Source: CAD feature listing. Evaluate the final solid. Frame: model axes, mm. A direction names the side the tool comes from. Coordinates: 2 decimals unless noted, no trailing zeros. Write each loop counter-clockwise with the first axis right and the second up, starting at its lowest first coordinate (ties: lowest second). Pieces come first, ordered by that corner, then holes. Notation, with made-up numbers: M 26,-31.5 L 73,-31.5 A18 ccw 73,-26.5 Z; hole C 34.25,17 d6. An arc over 180 degrees is marked long. Write item = value, one per line. Start each with the question number.
1. Access query for faces 5 (the face through (-40.52, 24.54, 33.99)), 6 (the face through (-40.52, 66.04, 33.99)), 7 (the face through (-36.61, 44.94, 34.79)), 8 (the face through (-91, 89, 30)), 9 (the face through (-100, 67, 30)). Directions: +Z, -Z, +X, -X, +Y, -Y. A direction counts if a zero-diameter tool reaches every point of the face in a straight line with its end or side. Return the directions, or none.
2. Pin query (flat end, axial travel): pin 1 Ø4 at (y, z) = (65, 25.5) entering from -X; pin 2 Ø10 at (x, y) = (-74, 22) entering from +Z; pin 3 Ø5 at (x, z) = (-90, 25.5) entering from +Y. Return the tip coordinate at first contact, or that it passes through.
3. Section query A-A (y = 10). Output: boundary loops of the cut face in (x, z).
4. Pull-direction query (Z, two-part tool) for faces 1 (the face through (-100.465, 30.344, 34.553)), 2 (the face through (-100, 28, 44.45)), 3 (the face through (-40, 68.5, 28)), 4 (the face through (-100.465, 25.776, 25.153)); classes: pulls with the +Z half, pulls with the -Z half, needs draft (parallel to the pull), parting line crosses it, or undercut.
5. Section query C-C (x = -100.5). Output: boundary loops of the cut face in (y, z).
6. Section query B-B (x = 10). Output: boundary loops of the cut face in (y, z).
7. Section query D-D (z = 24.45). Give the number of separate pieces and of enclosed holes in the cut face, then the cut area to 3 significant figures.
8. Line query: line 1 along Y through (x, z) = (10, 14.2); line 2 along Y through (x, z) = (-34, 31.5); line 3 along X through (y, z) = (87.75, 24.45). Output: solid intervals per line, ascending.
```python
from build123d import *

# Parameters (mm, degrees)
SKETCH169_R                = 2.34
EXTRUDE089_DEPTH           = 20
SKETCH168_W                = 10
SKETCH168_H                = 30
EXTRUDE088_DEPTH           = 5
EXTRUDE088_PLACEMENT_ANGLE = 90
CUT055_PLACEMENT_ANGLE     = 90
SKETCH165_R                = 2.34
EXTRUDE085_DEPTH           = 20
SKETCH164_W                = 10
SKETCH164_H                = 30
EXTRUDE084_DEPTH           = 5
EXTRUDE084_PLACEMENT_ANGLE = 90
SKETCH082_R                = 2.21
EXTRUDE103_DEPTH           = 10
SKETCH081_R                = 2.21
EXTRUDE102_DEPTH           = 10
SKETCH080_W                = 12
SKETCH080_H                = 26.01178
EXTRUDE101_DEPTH           = 5
SKETCH079_R                = 2.21
EXTRUDE100_DEPTH           = 10
SKETCH078_R                = 2.21
EXTRUDE099_DEPTH           = 10
SKETCH077_W                = 12
SKETCH077_H                = 26.01178
EXTRUDE098_DEPTH           = 5
SKETCH167_R                = 2.34
EXTRUDE087_DEPTH           = 20
SKETCH166_W                = 10
SKETCH166_H                = 30
EXTRUDE086_DEPTH           = 5
EXTRUDE086_PLACEMENT_ANGLE = 90
CUT052_PLACEMENT_ANGLE     = 90
SKETCH163_R                = 2.34
EXTRUDE083_DEPTH           = 20
SKETCH162_W                = 10
SKETCH162_H                = 30
EXTRUDE082_DEPTH           = 5
EXTRUDE082_PLACEMENT_ANGLE = 90
SKETCH016_R                = 2.005
EXTRUDE077_DEPTH           = 20
EXTRUDE076_DEPTH           = 20
EXTRUDE075_DEPTH           = 20
SKETCH161_W                = 10
SKETCH161_H                = 27.36
EXTRUDE182_DEPTH           = 70
SKETCH075_R                = 2.9
EXTRUDE091_DEPTH           = 50
SKETCH074_W                = 130
SKETCH074_H                = 90
EXTRUDE090_DEPTH           = 2


with BuildPart() as tornillos050:
    # Sketch169 (on Face6 of Extrude088) → Extrude089 (new body)
    with BuildSketch(Plane(origin=(-101, -107, 0), x_dir=(0, -1, 0), z_dir=(-1, 0, 0))):
        with Locations((-135.006037, 30)):
            Circle(SKETCH169_R)
        with Locations((-135.008375, 20)):
            Circle(SKETCH169_R)
    extrude(amount=EXTRUDE089_DEPTH)


with BuildPart() as tornillos050_1:
    # Extrude089 placement: moved
    add(tornillos050.part.moved(Location((17, 0, 0))))


with BuildPart() as soporte016:
    # Sketch168 → Extrude088 (new body)
    with BuildSketch(Plane.XZ):
        with Locations((-135, 25)):
            Rectangle(SKETCH168_W, SKETCH168_H)
    extrude(amount=EXTRUDE088_DEPTH)


with BuildPart() as soporte016_1:
    # Extrude088 placement: moved
    add(soporte016.part.moved(Location((-96, -107, 0))).rotate(Axis((-96, -107, 0), (0, 0, -1)), EXTRUDE088_PLACEMENT_ANGLE))

    # Cut055: cut Tornillos050
    add(tornillos050_1.part, mode=Mode.SUBTRACT)


with BuildPart() as soporte016_2:
    # Cut055 placement: moved
    add(soporte016_1.part.moved(Location((-119, -12, -3))).rotate(Axis((-119, -12, -3), (0, 0, -1)), CUT055_PLACEMENT_ANGLE))


with BuildPart() as tornillos048:
    # Sketch165 (on Face6 of Extrude084) → Extrude085 (new body)
    with BuildSketch(Plane(origin=(-101, -107, 0), x_dir=(0, -1, 0), z_dir=(-1, 0, 0))):
        with Locations((-135.006037, 30)):
            Circle(SKETCH165_R)
        with Locations((-135.008375, 20)):
            Circle(SKETCH165_R)
    extrude(amount=EXTRUDE085_DEPTH)


with BuildPart() as tornillos048_1:
    # Extrude085 placement: moved
    add(tornillos048.part.moved(Location((17, 0, 0))))


with BuildPart() as soporte015:
    # Sketch164 → Extrude084 (new body)
    with BuildSketch(Plane.XZ):
        with Locations((-135, 25)):
            Rectangle(SKETCH164_W, SKETCH164_H)
    extrude(amount=EXTRUDE084_DEPTH)


with BuildPart() as soporte015_1:
    # Extrude084 placement: moved
    add(soporte015.part.moved(Location((-96, -107, 0))).rotate(Axis((-96, -107, 0), (0, 0, -1)), EXTRUDE084_PLACEMENT_ANGLE))

    # Cut054: cut Tornillos048
    add(tornillos048_1.part, mode=Mode.SUBTRACT)


with BuildPart() as soporte015_2:
    # Cut054 placement: moved
    add(soporte015_1.part.moved(Location((-2, 34, -3))))


with BuildPart() as extrude103:
    # Sketch082 → Extrude103 (new body)
    with BuildSketch(Plane.XZ):
        with Locations((-30.242167, 20.01615)):
            Circle(SKETCH082_R)
    extrude(amount=EXTRUDE103_DEPTH)


with BuildPart() as extrude103_1:
    # Extrude103 placement: moved
    add(extrude103.part.moved(Location((-9.8, 5, -14.82))))


with BuildPart() as extrude102:
    # Sketch081 → Extrude102 (new body)
    with BuildSketch(Plane.XZ):
        with Locations((-30.242167, 20.01615)):
            Circle(SKETCH081_R)
    extrude(amount=EXTRUDE102_DEPTH)


with BuildPart() as extrude102_1:
    # Extrude102 placement: moved
    add(extrude102.part.moved(Location((-9.8, 3, 2.68))))


with BuildPart() as cut059:
    # Sketch080 → Extrude101 (new body)
    with BuildSketch(Plane.XZ):
        with Locations((-39.733391, 13.00589)):
            Rectangle(SKETCH080_W, SKETCH080_H)
    extrude(amount=EXTRUDE101_DEPTH)

    # Cut058: cut Extrude102
    add(extrude102_1.part, mode=Mode.SUBTRACT)

    # Cut059: cut Extrude103
    add(extrude103_1.part, mode=Mode.SUBTRACT)


with BuildPart() as cut059_1:
    # Cut059 placement: moved
    add(cut059.part.moved(Location((0, 68.5, 6))))


with BuildPart() as extrude100:
    # Sketch079 → Extrude100 (new body)
    with BuildSketch(Plane.XZ):
        with Locations((-30.242167, 20.01615)):
            Circle(SKETCH079_R)
    extrude(amount=EXTRUDE100_DEPTH)


with BuildPart() as extrude100_1:
    # Extrude100 placement: moved
    add(extrude100.part.moved(Location((-9.8, 5, -14.82))))


with BuildPart() as extrude099:
    # Sketch078 → Extrude099 (new body)
    with BuildSketch(Plane.XZ):
        with Locations((-30.242167, 20.01615)):
            Circle(SKETCH078_R)
    extrude(amount=EXTRUDE099_DEPTH)


with BuildPart() as extrude099_1:
    # Extrude099 placement: moved
    add(extrude099.part.moved(Location((-9.8, 3, 2.68))))


with BuildPart() as cut057:
    # Sketch077 → Extrude098 (new body)
    with BuildSketch(Plane.XZ):
        with Locations((-39.733391, 13.00589)):
            Rectangle(SKETCH077_W, SKETCH077_H)
    extrude(amount=EXTRUDE098_DEPTH)

    # Cut056: cut Extrude099
    add(extrude099_1.part, mode=Mode.SUBTRACT)

    # Cut057: cut Extrude100
    add(extrude100_1.part, mode=Mode.SUBTRACT)


with BuildPart() as cut057_1:
    # Cut057 placement: moved
    add(cut057.part.moved(Location((0, 27, 6))))


with BuildPart() as tornillos049:
    # Sketch167 (on Face6 of Extrude086) → Extrude087 (new body)
    with BuildSketch(Plane(origin=(-101, -107, 0), x_dir=(0, -1, 0), z_dir=(-1, 0, 0))):
        with Locations((-135.006037, 30)):
            Circle(SKETCH167_R)
        with Locations((-135.008375, 20)):
            Circle(SKETCH167_R)
    extrude(amount=EXTRUDE087_DEPTH)


with BuildPart() as tornillos049_1:
    # Extrude087 placement: moved
    add(tornillos049.part.moved(Location((17, 0, 0))))


with BuildPart() as soporte013:
    # Sketch166 → Extrude086 (new body)
    with BuildSketch(Plane.XZ):
        with Locations((-135, 25)):
            Rectangle(SKETCH166_W, SKETCH166_H)
    extrude(amount=EXTRUDE086_DEPTH)


with BuildPart() as soporte013_1:
    # Extrude086 placement: moved
    add(soporte013.part.moved(Location((-96, -107, 0))).rotate(Axis((-96, -107, 0), (0, 0, -1)), EXTRUDE086_PLACEMENT_ANGLE))

    # Cut052: cut Tornillos049
    add(tornillos049_1.part, mode=Mode.SUBTRACT)


with BuildPart() as soporte013_2:
    # Cut052 placement: moved
    add(soporte013_1.part.moved(Location((-119, -95, -3))).rotate(Axis((-119, -95, -3), (0, 0, -1)), CUT052_PLACEMENT_ANGLE))


with BuildPart() as tornillos047:
    # Sketch163 (on Face6 of Extrude082) → Extrude083 (new body)
    with BuildSketch(Plane(origin=(-101, -107, 0), x_dir=(0, -1, 0), z_dir=(-1, 0, 0))):
        with Locations((-135.006037, 30)):
            Circle(SKETCH163_R)
        with Locations((-135.008375, 20)):
            Circle(SKETCH163_R)
    extrude(amount=EXTRUDE083_DEPTH)


with BuildPart() as tornillos047_1:
    # Extrude083 placement: moved
    add(tornillos047.part.moved(Location((17, 0, 0))))


with BuildPart() as soporte014:
    # Sketch162 → Extrude082 (new body)
    with BuildSketch(Plane.XZ):
        with Locations((-135, 25)):
            Rectangle(SKETCH162_W, SKETCH162_H)
    extrude(amount=EXTRUDE082_DEPTH)


with BuildPart() as soporte014_1:
    # Extrude082 placement: moved
    add(soporte014.part.moved(Location((-96, -107, 0))).rotate(Axis((-96, -107, 0), (0, 0, -1)), EXTRUDE082_PLACEMENT_ANGLE))

    # Cut053: cut Tornillos047
    add(tornillos047_1.part, mode=Mode.SUBTRACT)


with BuildPart() as soporte014_2:
    # Cut053 placement: moved
    add(soporte014_1.part.moved(Location((-2, 0, -3))))


with BuildPart() as tornillo018:
    # Sketch016 → Extrude077 (new body)
    with BuildSketch(Plane.XY.offset(45.913223)):
        with Locations((-84.962639, 67.504814)):
            Circle(SKETCH016_R)
    extrude(amount=EXTRUDE077_DEPTH)


with BuildPart() as tornillo018_1:
    # Extrude077 placement: moved
    add(tornillo018.part.moved(Location((46.5, -21.8, -26))))


with BuildPart() as tornillo017:
    # Sketch016 → Extrude076 (new body)
    with BuildSketch(Plane.XY.offset(45.913223)):
        with Locations((-84.962639, 67.504814)):
            Circle(SKETCH016_R)
    extrude(amount=EXTRUDE076_DEPTH)


with BuildPart() as tornillo017_1:
    # Extrude076 placement: moved
    add(tornillo017.part.moved(Location((23.6, -21.8, -25.9))))


with BuildPart() as tornillo016:
    # Sketch016 → Extrude075 (new body)
    with BuildSketch(Plane.XY.offset(45.913223)):
        with Locations((-84.962639, 67.504814)):
            Circle(SKETCH016_R)
    extrude(amount=EXTRUDE075_DEPTH)


with BuildPart() as tornillo016_1:
    # Extrude075 placement: moved
    add(tornillo016.part.moved(Location((0, -21.8, -26))))


with BuildPart() as obj1:
    # Sketch161 → Extrude182 (new body)
    with BuildSketch(Plane.YZ):
        with Locations((-10.400922, 22.215275)):
            Rectangle(SKETCH161_W, SKETCH161_H)
    extrude(amount=EXTRUDE182_DEPTH)


with BuildPart() as obj1_1:
    # Extrude182 placement: moved
    add(obj1.part.moved(Location((-95, 56.4, -0.3))))

    # Cut107: cut Tornillo016
    add(tornillo016_1.part, mode=Mode.SUBTRACT)

    # Cut044: cut Tornillo017
    add(tornillo017_1.part, mode=Mode.SUBTRACT)

    # Cut045: cut Tornillo018
    add(tornillo018_1.part, mode=Mode.SUBTRACT)


with BuildPart() as obj1_2:
    # Cut045 placement: moved
    add(obj1_1.part.moved(Location((0, 0, -0.3))))


with BuildPart() as tornillos051:
    # Sketch075 (on Face6 of Extrude090) → Extrude091 (new body)
    with BuildSketch(Plane.XY.offset(2)):
        with Locations((120, 80.020506)):
            Circle(SKETCH075_R)
        with Locations((120, 45.010253)):
            Circle(SKETCH075_R)
        with Locations((120, 10)):
            Circle(SKETCH075_R)
    extrude(amount=EXTRUDE091_DEPTH)


with BuildPart() as tornillos051_1:
    # Extrude091 placement: moved
    add(tornillos051.part.moved(Location((0, 0, -31))))


with BuildPart() as obj2:
    # Sketch074 → Extrude090 (new body)
    with BuildSketch(Plane.XY):
        with Locations((65, 45)):
            Rectangle(SKETCH074_W, SKETCH074_H)
    extrude(amount=EXTRUDE090_DEPTH)

    # Cut047: cut Tornillos051
    add(tornillos051_1.part, mode=Mode.SUBTRACT)


with BuildPart() as obj2_1:
    # Cut047 placement: moved
    add(obj2.part.moved(Location((-110, 0, 6))))

    # Fusion059: union obj1
    add(obj1_2.part)

    # Fusion060: union Soporte014
    add(soporte014_2.part)

    # Fusion061: union Soporte013
    add(soporte013_2.part)

    # Fusion062: union Cut057
    add(cut057_1.part)

    # Fusion023: union Cut059
    add(cut059_1.part)

    # Fusion024: union Soporte015
    add(soporte015_2.part)

    # Fusion025: union Soporte016
    add(soporte016_2.part)


with BuildPart() as obj2_2:
    # Fusion025 placement: moved
    add(obj2_1.part.moved(Location((0, 0, 7.45))))


solid = obj2_2.part
```
Results are:
q1.face_5 = -Y
q1.face_6 = +Y
q1.face_7 = +Z
q1.face_8 = +Z, +X, -X, +Y
q1.face_9 = +Z, -X, +Y
q2.pin_1 = -103
q2.pin_2 = 15.45
q2.pin_3 = 89
q3.outline = M -110,13.45 L 7.1,13.45 L 7.1,15.45 L -110,15.45 Z; M 12.9,13.45 L 20,13.45 L 20,15.45 L 12.9,15.45 Z
q4.face_1 = undercut
q4.face_2 = pulls with the +Z half
q4.face_3 = needs draft
q4.face_4 = undercut
q5.outline = M 0,13.45 L 90,13.45 L 90,15.45 L 67,15.45 L 67,44.45 L 57,44.45 L 57,15.45 L 33,15.45 L 33,44.45 L 23,44.45 L 23,15.45 L 0,15.45 Z; hole C 28.01,24.45 d4.68; hole C 28.01,34.45 d4.68; hole C 62.01,24.45 d4.68; hole C 62.01,34.45 d4.68
q6.outline = M 0,13.45 L 7.1,13.45 L 7.1,15.45 L 0,15.45 Z; M 12.9,13.45 L 42.11,13.45 L 42.11,15.45 L 12.9,15.45 Z; M 47.91,13.45 L 77.12,13.45 L 77.12,15.45 L 47.91,15.45 Z; M 82.92,13.45 L 90,13.45 L 90,15.45 L 82.92,15.45 Z
q7.separate_pieces = 11
q7.enclosed_holes = 0
q7.area = 926 mm^2
q8.line_1 = 0 to 7.1, 12.9 to 42.11, 47.91 to 77.12, 82.92 to 90
q8.line_2 = 22 to 27, 41 to 51, 63.5 to 68.5
q8.line_3 = -96 to -93.33, -88.65 to -86
